Work out the finished part from the listing and answer in its coordinate system (mm). A direction names the side the tool comes from. Round coordinates to 2 decimals unless told otherwise and drop trailing zeros. Write each loop counter-clockwise with the first axis right and the second up, starting at its lowest first coordinate (ties: lowest second). Pieces come first, ordered by that corner, then holes.
1. Find section A-A (z = 15.25). Write down the section's boundary in (x, y).
2. Flat-ended cylindrical pins translate along their axes: pin 1 Ø1.5 at (y, z) = (30.5, 2) entering from -X; pin 2 Ø1 at (y, z) = (60, 9.5) entering from +X; pin 3 Ø10 at (x, y) = (47.5, 26) entering from +Z. Find the tip coordinate at first contact, or state that the pin passes through.
3. Find section B-B (x = 45.5). Write down the section's boundary in (y, z).
4. A tool of negligible diameter and unlimited length cuts with its end or side. For faces 4 (the face through (92.297, 72.325, 9.319)), 5 (the face through (45, 31.043, 3)), 6 (the face through (50.6, 40.9, 19.14)), from which of +Z, -Z, +X, -X, +Y, -Y can it reach the whole face along a straight path? Write none if from no direction.
5. Determine the mould class of faces 1 (the face through (9.825, 72.325, 6.935)), 2 (the face through (49, 0, 10)), 3 (the face through (90, 30, 11)) for opening direction Y: pulls with the +Y half, pulls with the -Y half, needs draft (parallel to the pull), parting line crosses it, or undercut.
6. Find section D-D (y = 36.5). Write down the section's boundary in (x, z).
7. Find section C-C (x = 14). Write down the section's boundary in (y, z).
8. Straight lines are drawn through the part: probe 1 along Y at (x, z) = (77, 8.5); probe 2 along X at (y, z) = (28.5, 3); probe 3 along Y at (x, z) = (94.5, 16.25). For each, find the intervals that lie inside material, in ascending order.
Autodesk Inventor part; units mm, degrees
ref_plane "YZ Plane" through (0, 0, 0) normal (1, 0, 0) x (0, 1, 0)
ref_plane "XZ Plane" through (0, 0, 0) normal (0, 1, 0) x (-1, 0, 0)
ref_plane "XY Plane" through (0, 0, 0) normal (0, 0, 1) x (1, 0, 0)
sketch "Sketch1" plane through (0, 0, 0) normal (0, 0, 1) x (1, 0, 0)
  line L0 (0, 60) -> (0, 0)
  line L1 (0, 0) -> (100, 0)
  line L2 (100, 0) -> (100, 60)
  line L3 (100, 60) -> (0, 60)
extrude "Extrusion1" add sketch "Sketch1" along normal blind 20
sketch "Sketch2" plane through (0, 0, 20) normal (0, 0, 1) x (1, 0, 0)
  line L0 (10, 40) -> (90, 40)
  line L1 (90, 40) -> (90, 20)
  line L2 (90, 20) -> (10, 20)
  line L3 (10, 20) -> (10, 40)
  line L4 (100, 60) -> (0, 60)
  line L5 (0, 0) -> (100, 0)
  line L6 (100, 0) -> (100, 60)
  line L7 (0, 60) -> (0, 0)
extrude "Extrusion2" cut sketch "Sketch2" against normal blind 15 contours L0 L1 L2 L3
sketch "Sketch3" plane through (0, 0, 20) normal (0, 0, 1) x (1, 0, 0)
  line L0 (38.6013, 31.0426) -> (51.4646, 31.0426)
  line L1 (51.4646, 31.0426) -> (51.4646, 28.004)
  line L2 (51.4646, 28.004) -> (38.6013, 28.004)
  line L3 (38.6013, 28.004) -> (38.6013, 31.0426)
  point P0 (0, 0)
extrude "Extrusion3" cut sketch "Sketch3" against normal through all
sketch "Sketch4" plane through (0, 60, 0) normal (0, 1, 0) x (1, 0, 0)
  line L0 (0, 0) -> (0, -20)
  line L1 (100, 0) -> (100, -20)
  circle A0 centre (10.2828, -8.9975) radius 2.1128
  circle A1 centre (90.2822, -8.6847) radius 2.1128
  dimension "d18" = 80
extrude "Extrusion4" add sketch "Sketch4" along normal blind 25
sketch "Sketch5" plane through (0, 60, 0) normal (0, 1, 0) x (1, 0, 0)
  circle A0 centre (10.2828, -8.9975) radius 2.1128
  line L0 (97.4061, -6.1607) -> (97.5, -6.1584)
  line L1 (10.2828, -5.156) -> (10.2828, -8.9975)
  point P0 (0, 0)
fillet "Fillet1" radius 3 13 edges at (50, 60, 20) (100, 30, 20) (100, 60, 10) (100, 30, 0) (50, 60, 0) (50, 0, 20) (50, 20, 20) (50, 40, 20) (10, 30, 20) (90, 30, 20) (0, 30, 20) (0, 30, 0) (50, 0, 0)
properties part number "part3nn" material "Polyethylene, High Density"
Worked answers:
1. outline: (0, 0) - (100, 0) - (100, 57) arc R3 ccw to (97, 60) - (0, 60) - close; hole (10, 20) - (90, 20) - (90, 40) - (10, 40) - close
2. pin 1: stops at x = 0.01
2. pin 2: stops at x = 98.66
2. pin 3: stops at z = 5
3. outline: (0, 3) arc R3 ccw to (3, 0) - (28, 0) - (28, 5) - (20, 5) - (20, 17) arc R3 ccw to (17, 20) - (3, 20) arc R3 ccw to (0, 17) - close; (31.04, 0) - (57, 0) arc R3 ccw to (60, 3) - (60, 17) arc R3 ccw to (57, 20) - (43, 20) arc R3 ccw to (40, 17) - (40, 5) - (31.04, 5) - close
4. face 4: +Y
4. face 5: +Z, -Z
4. face 6: +Z
5. face 1: needs draft
5. face 2: pulls with the -Y half
5. face 3: undercut
6. outline: (0, 3) arc R3 ccw to (3, 0) - (97, 0) arc R3 ccw to (100, 3) - (100, 17) arc R3 ccw to (97, 20) - (93, 20) arc R3 ccw to (90, 17) - (90, 5) - (10, 5) - (10, 17) arc R3 ccw to (7, 20) - (3, 20) arc R3 ccw to (0, 17) - close
7. outline: (0, 3) arc R3 ccw to (3, 0) - (57, 0) arc R3 ccw to (60, 3) - (60, 17) arc R3 ccw to (57, 20) - (43, 20) arc R3 ccw to (40, 17) - (40, 5) - (20, 5) - (20, 17) arc R3 ccw to (17, 20) - (3, 20) arc R3 ccw to (0, 17) - close
8. probe 1: y = 0 to 20, 40 to 60
8. probe 2: x = 0 to 38.6, 51.46 to 100
8. probe 3: y = 0 to 60
